from build123d import *

# Parameters (mm, degrees)
F0_W     = 2057.4
F0_H     = 406.4
F0_W_2   = 1000.125
F0_H_2   = 368.3
F1_DEPTH = 508
F2_W     = 101.6
F2_H     = 19.05
F3_DEPTH = 2057.401
F4_W     = 2057.4
F4_H     = 387.35
F5_DEPTH = 19.05
F6_W     = 152.4
F6_H     = 1009.65
F6_H_2   = 1000.125
F7_DEPTH = 19.05
F8_W     = 1000.125
F8_H     = 368.3
F8_W_2   = 962.025
F8_H_2   = 330.2
F9_DEPTH = 76.2
F10_SIZE = 19.05


with BuildPart() as f1:
    # F0 (on Right) → F1 (new body)
    with BuildSketch(Plane.YZ):
        Rectangle(F0_W, F0_H)
        with Locations((-509.5875, 0)):
            Rectangle(F0_W_2, F0_H_2, mode=Mode.SUBTRACT)
        with Locations((509.5875, 0)):
            Rectangle(F0_W_2, F0_H_2, mode=Mode.SUBTRACT)
    extrude(amount=-F1_DEPTH)

    # F2 (on face) → F3 (cut, through all)
    with BuildSketch(Plane.XZ.offset(1028.7)):
        with Locations((-457.2, 193.675)):
            Rectangle(F2_W, F2_H)
    extrude(amount=-F3_DEPTH, mode=Mode.SUBTRACT)

    # F4 (on face) → F5 (join)
    with BuildSketch(Plane(origin=(-508, 0, 0), x_dir=(0, -1, 0), z_dir=(-1, 0, 0))):
        with Locations((0, -9.525)):
            Rectangle(F4_W, F4_H)
    extrude(amount=F5_DEPTH)

    # F6 (on face) → F7 (join)
    with BuildSketch(Plane(origin=(0, 0, 184.15), x_dir=(1, 0, 0), z_dir=(0, 0, -1))):
        with Locations((-431.8, -504.825)):
            Rectangle(F6_W, F6_H)
        with Locations((-431.8, 509.5875)):
            Rectangle(F6_W, F6_H_2)
    extrude(amount=F7_DEPTH)

    # F8 (on face) → F9 (join)
    with BuildSketch(Plane.YZ):
        with Locations((-509.5875, 0)):
            Rectangle(F8_W, F8_H)
        with Locations((-509.5875, 0)):
            Rectangle(F8_W_2, F8_H_2, mode=Mode.SUBTRACT)
        with Locations((509.5875, 0)):
            Rectangle(F8_W, F8_H)
        with Locations((509.5875, 0)):
            Rectangle(F8_W_2, F8_H_2, mode=Mode.SUBTRACT)
    extrude(amount=-F9_DEPTH)

    # F10
    f10_edges = [f1.edges().sort_by_distance(p)[0] for p in [
        (0, -509.5875, 165.1),
        (0, -990.6, 0),
        (0, -509.5875, -165.1),
        (0, -28.575, 0),
        (0, 509.5875, -165.1),
        (0, 28.575, 0),
        (0, 509.5875, 165.1),
        (0, 990.6, 0),
    ]]
    chamfer(f10_edges, length=F10_SIZE)


solid = f1.part
Geometry: final body of the model. Coordinates: model frame, mm. A direction names the side the tool comes from. Round coordinates to 2 decimals unless told otherwise and drop trailing zeros. Loops run counter-clockwise (first coordinate to the right, second up) from the corner with the lowest first, then second, coordinate; pieces in that order, holes last.
Q1. Pull-direction query (X, two-part tool) for faces 6 (the flat face through (-289, 9.525, -3)), 7 (the flat face through (-47, 503, -165.1)); classes: released by +X, released by -X, zero draft, split by the parting line, or undercut.
Q2. Section A-A on x = -337. Return loops of the section in (y, z) (3 decimals), plus the area to 3 significant figures.
Q3. Section B-B on z = 124.5. Return loops of the section in (x, y) (3 decimals), plus the area to 3 significant figures.
Q4. Section C-C on y = -879. Return loops of the section in (x, z), plus the area to 3 significant figures.
Q5. Section D-D on x = -447. Return loops of the section in (y, z) (3 decimals), plus the area to 3 significant figures.
Q6. Access query for faces 1 (the flat face through (-47, -990.6, -2)), 2 (the flat face through (-76.2, -660, -176)), 3 (the flat face through (-260, -1028.7, -3)), 4 (the flat face through (-260, 14, -203.2)), 5 (the flat face through (-468, -14, 184.15)). Directions: +Z, -Z, +X, -X, +Y, -Y. A direction counts if a zero-diameter tool reaches every point of the face in a straight line with its end or side. Return the directions, or none.
Q7. Pin query (flat end, axial travel): P1, Ø8, axis at y = 368, z = 125, coming from the +X side; P2, Ø1.5, axis at x = -447, y = -44.5, coming from the +Z side. Return the tip coordinate at first contact, or that it passes through.
Q8. Material intervals for L1, parallel to Y at x = -191, z = -5.5 (3 decimals); L2, parallel to Y at x = -43, z = 27 (3 decimals); L3, parallel to Z at x = -314.5, y = -505, sorted ascending.
Evaluation:
1. face 6: undercut
1. face 7: zero draft
2. outline: (-1028.7, -203.2) - (1028.7, -203.2) - (1028.7, 203.2) - (-1028.7, 203.2) - close; hole (-1009.65, -184.15) - (-9.525, -184.15) - (-9.525, 184.15) - (-1009.65, 184.15) - close; hole (9.525, -184.15) - (1009.65, -184.15) - (1009.65, 184.15) - (9.525, 184.15) - close
2. area: 99,400 mm2
3. outline: (-527.05, -1028.7) - (0, -1028.7) - (0, -1009.65) - (-19.05, -990.6) - (-76.2, -990.6) - (-76.2, -1009.65) - (-508, -1009.65) - (-508, -9.525) - (-76.2, -9.525) - (-76.2, -28.575) - (-19.05, -28.575) - (0, -9.525) - (0, 9.525) - (-19.05, 28.575) - (-76.2, 28.575) - (-76.2, 9.525) - (-508, 9.525) - (-508, 1009.65) - (-76.2, 1009.65) - (-76.2, 990.6) - (-19.05, 990.6) - (0, 1009.65) - (0, 1028.7) - (-527.05, 1028.7) - close
3. area: 73,300 mm2
4. outline: (-527.05, -203.2) - (0, -203.2) - (0, -184.15) - (-19.05, -165.1) - (-76.2, -165.1) - (-76.2, -184.15) - (-508, -184.15) - (-508, 165.1) - (-355.6, 165.1) - (-355.6, 184.15) - (-76.2, 184.15) - (-76.2, 165.1) - (-19.05, 165.1) - (0, 184.15) - (0, 203.2) - (-406.4, 203.2) - (-406.4, 184.15) - (-527.05, 184.15) - close
4. area: 30,200 mm2
5. outline: (-1028.7, -203.2) - (1028.7, -203.2) - (1028.7, 184.15) - (-1028.7, 184.15) - close; hole (-1009.65, -184.15) - (-9.525, -184.15) - (-9.525, 165.1) - (-1009.65, 165.1) - close; hole (9.525, -184.15) - (1009.65, -184.15) - (1009.65, 165.1) - (9.525, 165.1) - close
5. area: 98,300 mm2
6. face 1: +X
6. face 2: none
6. face 3: +Z, -Z, +X, -X, -Y
6. face 4: -Z, +X, -X, +Y, -Y
6. face 5: +Z, -X, +Y, -Y
7. P1: stops at x = -508
7. P2: stops at z = 184.15
8. L1: y = -1028.7 to -1009.65, -9.525 to 9.525, 1009.65 to 1028.7
8. L2: y = -1028.7 to -990.6, -28.575 to 28.575, 990.6 to 1028.7
8. L3: z = -203.2 to -184.15, 184.15 to 203.2
